Autodesk Inventor part; units mm, degrees
ref_plane "YZ Plane" through (0, 0, 0) normal (1, 0, 0) x (0, 1, 0)
ref_plane "XZ Plane" through (0, 0, 0) normal (0, 1, 0) x (-1, 0, 0)
ref_plane "XY Plane" through (0, 0, 0) normal (0, 0, 1) x (1, 0, 0)
sketch "Sketch1" plane through (0, 0, 0) normal (0, 0, 1) x (1, 0, 0)
  line L0 (0, 0) -> (101.6, 0)
  line L1 (101.6, 0) -> (101.6, 44.45)
  line L2 (101.6, 44.45) -> (0, 44.45)
  line L3 (0, 44.45) -> (0, 0)
  dimension "d0" = 101.6
  dimension "d1" = 44.45
extrude "Extrusion1" add sketch "Sketch1" along normal blind 25.4
sketch "Sketch2" plane through (0, 0, 25.4) normal (0, 0, 1) x (1, 0, 0)
  line L0 (0, 0) -> (101.6, 0)
  line L1 (101.6, 0) -> (101.6, 44.45)
  line L2 (101.6, 44.45) -> (0, 44.45)
  line L3 (0, 44.45) -> (0, 0)
  line L4 (3.175, 41.275) -> (98.425, 41.275)
  line L5 (98.425, 41.275) -> (98.425, 3.175)
  line L6 (98.425, 3.175) -> (3.175, 3.175)
  line L7 (3.175, 3.175) -> (3.175, 41.275)
  dimension "d4" = 3.175
extrude "Extrusion2" cut sketch "Sketch2" against normal blind 12.7
sketch "Sketch3" plane through (0, 0, 0) normal (0, 0, -1) x (-1, 0, 0)
  line L0 (0, 44.45) -> (0, 0)
  line L1 (-101.6, 44.45) -> (0, 44.45)
  line L2 (-101.6, 0) -> (-101.6, 44.45)
  point P0 (-76.2, 22.225)
  point P1 (-25.4, 22.225)
  dimension "d7" = 50.8
  dimension "d8" = 25.4
  dimension "d9" = 25.4
  dimension "d10" = 22.225
hole "Hole1" at (76.2, 22.225, 0) at (25.4, 22.225, 0) direction (0, 0, 1) diameter 4.9784 end through all
properties part number "Endcaps"
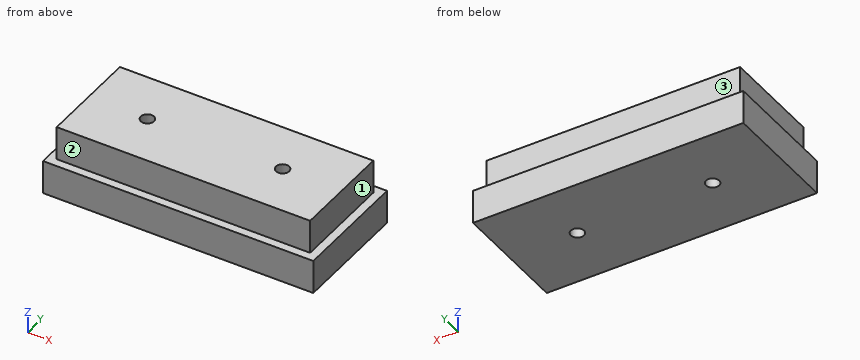
Input: part model. Units: mm. Frame: model coordinates. Face numbers are marked on the shaded views. A direction names the side the tool comes from. Give positions to 0.01 mm unless a question says otherwise; leave off trailing zeros. Loops run counter-clockwise (first coordinate to the right, second up) from the corner with the lowest first, then second, coordinate; pieces in that order, holes last. Notation, with made-up numbers: M 21,55.5 L 79,55.5 A20 cw 79,92.5 Z; hole C -18,81 d5. An arc over 180 degrees is marked long. Answer as CSV lines item,"result". Start each with the question number.
1. Section A-A on x = 25.4. Return loops of the section in (y, z) (3 decimals), plus the area to 3 significant figures.
2. Line query: L1, parallel to Y at x = 25.4, z = 19.75 (3 decimals); L2, parallel to X at y = 21, z = 10; L3, parallel to Y at x = 29.5, z = 22.75 (3 decimals). Output: solid intervals per line, ascending.
3. Section C-C on y = 22.5. Return loops of the section in (x, z) (3 decimals).
4. Section D-D on x = 62.5. Return loops of the section in (y, z) (3 decimals).
5. Reachability of the marked faces 1, 2 and 3 from +Z, -Z, +X, -X, +Y, -Y: full face, straight path, thin tool, end or side. Return the list, or none.
6. Pin query (flat end, axial travel): P1, Ø14, axis at y = 17.5, z = 20, coming from the +X side (3 decimals); P2, Ø4, axis at x = 67, z = 17.5, coming from the -Y side (3 decimals); P3, Ø4, axis at x = 64, z = 19, coming from the +Y side (3 decimals). Return the tip coordinate at first contact, or that it passes through.
7. Section B-B on z = 18. Return loops of the section in (x, y) (3 decimals), plus the area to 3 significant figures.
Computed values:
1,outline,"M 0,0 L 19.736,0 L 19.736,25.4 L 3.175,25.4 L 3.175,12.7 L 0,12.7 Z; M 24.714,0 L 44.45,0 L 44.45,12.7 L 41.275,12.7 L 41.275,25.4 L 24.714,25.4 Z"
1,area,"922 mm²"
2,L1,"y = 3.175 to 19.736, 24.714 to 41.275"
2,L2,"x = 0 to 23.23, 27.57 to 74.03, 78.37 to 101.6"
2,L3,"y = 3.175 to 41.275"
3,outline,"M 0,0 L 22.926,0 L 22.926,25.4 L 3.175,25.4 L 3.175,12.7 L 0,12.7 Z; M 27.874,0 L 73.726,0 L 73.726,25.4 L 27.874,25.4 Z; M 78.674,0 L 101.6,0 L 101.6,12.7 L 98.425,12.7 L 98.425,25.4 L 78.674,25.4 Z"
4,outline,"M 0,0 L 44.45,0 L 44.45,12.7 L 41.275,12.7 L 41.275,25.4 L 3.175,25.4 L 3.175,12.7 L 0,12.7 Z"
5,face 1,"+Z, +X, +Y, -Y"
5,face 2,"+Z, +X, -X, -Y"
5,face 3,"+Z, +X, -X, +Y"
6,P1,"stops at x = 98.425"
6,P2,"stops at y = 3.175"
6,P3,"stops at y = 41.275"
7,outline,"M 3.175,3.175 L 98.425,3.175 L 98.425,41.275 L 3.175,41.275 Z; hole C 25.4,22.225 d4.978; hole C 76.2,22.225 d4.978"
7,area,"3,590 mm²"
